from build123d import *

# Parameters (mm, degrees)
BASE_START                                   = 59
BASE_PLATE_DEPTH                             = 5
BOLT_START                                   = 58.8
SKETCH2_R                                    = 1.7
BOLT_HOLES_CABLE_KIDNEY_DEPTH                = 5.4
CHEEK_START                                  = -36
CHEEK_X_DEPTH                                = 6
PIVOT_START                                  = -36
SKETCH4_R                                    = 17
PIVOT_BOSS_X_DEPTH                           = 6
CHEEK_START_2                                = 30
CHEEK_X_2_DEPTH                              = 6
PIVOT_START_2                                = 30
SKETCH6_R                                    = 17
PIVOT_BOSS_X_2_DEPTH                         = 6
JOURNAL_START                                = -37
SKETCH7_R                                    = 7.25
JOURNAL_BORES_DEPTH                          = 74
BACK_START                                   = -54
SKETCH8_W                                    = 72
SKETCH8_H                                    = 60.7
BACK_WALL_DEPTH                              = 4
PINION_START                                 = -55
SKETCH9_W                                    = 9.2
SKETCH9_H                                    = 45
PINION_NOTCH_DEPTH                           = 6
SERVO_START                                  = 0.55
SKETCH10_W                                   = 28.2
SKETCH10_H                                   = 58.7
SKETCH10_W_2                                 = 20.5
SKETCH10_H_2                                 = 41.5
SERVO_BULKHEAD_DEPTH                         = 5
TAB_START                                    = 0.35
SKETCH11_R                                   = 1.7
TAB_BOLT_HOLES_DEPTH                         = 5.4
TAB_START_2                                  = 2.85
TAB_NUT_POCKETS_DEPTH                        = 2.9
BULKHEAD_START                               = 0.35
BULKHEAD_CHAMFER_DEPTH                       = 5.4
HAND_START                                   = 0.35
SKETCH14_W                                   = 21.65
SKETCH14_H                                   = 13.8
HAND_FIX_BAR_OVER_THE_SERVO_WINDOW_SAW_DEPTH = 5.4


with BuildPart() as part:
    # Sketch1 → Base plate (new body)
    with BuildSketch(Plane(origin=(0, 0, 0), x_dir=(1, 0, 0), z_dir=(0, 1, 0)).offset(BASE_START)):
        with BuildLine():
            Line((-30, 54), (30, 54))
            ThreePointArc((30, 54), (34.242640687, 52.242640687), (36, 48))
            Line((36, 48), (36, -20))
            ThreePointArc((36, -20), (33.071067812, -27.071067812), (26, -30))
            Line((26, -30), (-26, -30))
            ThreePointArc((-26, -30), (-33.071067812, -27.071067812), (-36, -20))
            Line((-36, -20), (-36, 48))
            ThreePointArc((-36, 48), (-34.242640687, 52.242640687), (-30, 54))
        make_face()
    extrude(amount=BASE_PLATE_DEPTH)

    # Sketch2 → Bolt holes _ cable kidney (cut)
    with BuildSketch(Plane(origin=(0, 0, 0), x_dir=(1, 0, 0), z_dir=(0, 1, 0)).offset(BOLT_START)):
        with Locations(Location((-26, 44, 0), (0, 0, 90))):
            Circle(SKETCH2_R)
        with Locations(Location((-26, -22, 0), (0, 0, 90))):
            Circle(SKETCH2_R)
        with Locations(Location((26, 44, 0), (0, 0, 90))):
            Circle(SKETCH2_R)
        with Locations(Location((26, -22, 0), (0, 0, 90))):
            Circle(SKETCH2_R)
        with BuildLine():
            ThreePointArc((-35.238044383, 29.568230046), (0, 46), (35.238044383, 29.568230046))
            ThreePointArc((35.238044383, 29.568230046), (34.498503383, 21.115237729), (26.045511066, 21.854778729))
            ThreePointArc((26.045511066, 21.854778729), (0, 34), (-26.045511066, 21.854778729))
            ThreePointArc((-26.045511066, 21.854778729), (-34.498503383, 21.115237729), (-35.238044383, 29.568230046))
        make_face()
    extrude(amount=BOLT_HOLES_CABLE_KIDNEY_DEPTH, mode=Mode.SUBTRACT)


with BuildPart() as bolt_holes_cable_kidney_piece_1:
    # of the separate pieces the step leaves, piece 1, a body of its own (bolt_holes_cable_kidney_pieces)
    add(part.part.solids().sort_by_distance((-36, 59, 20))[0])



with BuildPart() as bolt_holes_cable_kidney_piece_2:
    # of the separate pieces the step leaves, piece 2, a body of its own (bolt_holes_cable_kidney_pieces)
    add(part.part.solids().sort_by_distance((-30, 59, -54))[0])


with BuildPart() as bolt_holes_cable_kidney_piece_1_1:
    add(bolt_holes_cable_kidney_piece_1.part)

    add(bolt_holes_cable_kidney_piece_2.part)  # Cheek -X merges Bolt holes _ cable kidney piece 2
    # Sketch3 → Cheek -X (add)
    with BuildSketch(Plane(origin=(0, 0, 0), x_dir=(0, 0, -1), z_dir=(1, 0, 0)).offset(CHEEK_START)):
        with BuildLine():
            Line((54, 63.8), (-22, 63.8))
            ThreePointArc((-22, 63.8), (-26.242640687, 65.557359313), (-28, 69.8))
            Line((-28, 69.8), (-28, 96.357864376))
            ThreePointArc((-28, 96.357864376), (-27.238795325, 100.1846987), (-25.071067812, 103.428932188))
            Line((-25.071067812, 103.428932188), (-11.622364452, 116.877635548))
            ThreePointArc((-11.622364452, 116.877635548), (-9.843658462, 118.217921148), (-7.764386256, 119.015910864))
            Line((-7.764386256, 119.015910864), (15.334171088, 124.346347174))
            ThreePointArc((15.334171088, 124.346347174), (16.004388899, 124.461463035), (16.683328128, 124.5))
            Line((16.683328128, 124.5), (54, 124.5))
            Line((54, 124.5), (54, 63.8))
        make_face()
    extrude(amount=CHEEK_X_DEPTH)

    # Sketch4 → Pivot boss -X (add)
    with BuildSketch(Plane(origin=(0, 0, 0), x_dir=(0, 0, -1), z_dir=(1, 0, 0)).offset(PIVOT_START)):
        with Locations((-14, 102.5)):
            Circle(SKETCH4_R)
    extrude(amount=PIVOT_BOSS_X_DEPTH)

    # Sketch5 → Cheek _X 2 (add)
    with BuildSketch(Plane(origin=(0, 0, 0), x_dir=(0, 0, -1), z_dir=(1, 0, 0)).offset(CHEEK_START_2)):
        with BuildLine():
            Line((54, 63.8), (-22, 63.8))
            ThreePointArc((-22, 63.8), (-26.242640687, 65.557359313), (-28, 69.8))
            Line((-28, 69.8), (-28, 96.357864376))
            ThreePointArc((-28, 96.357864376), (-27.238795325, 100.1846987), (-25.071067812, 103.428932188))
            Line((-25.071067812, 103.428932188), (-11.622364452, 116.877635548))
            ThreePointArc((-11.622364452, 116.877635548), (-9.843658462, 118.217921148), (-7.764386256, 119.015910864))
            Line((-7.764386256, 119.015910864), (15.334171088, 124.346347174))
            ThreePointArc((15.334171088, 124.346347174), (16.004388899, 124.461463035), (16.683328128, 124.5))
            Line((16.683328128, 124.5), (54, 124.5))
            Line((54, 124.5), (54, 63.8))
        make_face()
    extrude(amount=CHEEK_X_2_DEPTH)

    # Sketch6 → Pivot boss _X 2 (add)
    with BuildSketch(Plane(origin=(0, 0, 0), x_dir=(0, 0, -1), z_dir=(1, 0, 0)).offset(PIVOT_START_2)):
        with Locations((-14, 102.5)):
            Circle(SKETCH6_R)
    extrude(amount=PIVOT_BOSS_X_2_DEPTH)

    # Sketch7 → Journal bores (cut)
    with BuildSketch(Plane(origin=(0, 0, 0), x_dir=(0, 0, -1), z_dir=(1, 0, 0)).offset(JOURNAL_START)):
        with Locations(Location((-14, 102.5, 0), (0, 0, 180))):
            Circle(SKETCH7_R)
    extrude(amount=JOURNAL_BORES_DEPTH, mode=Mode.SUBTRACT)

    # Sketch8 → Back wall (add)
    with BuildSketch(Plane.XY.offset(BACK_START)):
        with Locations((0, 94.15)):
            Rectangle(SKETCH8_W, SKETCH8_H)
    extrude(amount=BACK_WALL_DEPTH)

    # Sketch9 → Pinion notch (cut)
    with BuildSketch(Plane.XY.offset(PINION_START)):
        with Locations((24.85, 103)):
            Rectangle(SKETCH9_W, SKETCH9_H)
    extrude(amount=PINION_NOTCH_DEPTH, mode=Mode.SUBTRACT)

    # Sketch10 → Servo bulkhead (add)
    with BuildSketch(Plane(origin=(0, 0, 0), x_dir=(0, 0, -1), z_dir=(1, 0, 0)).offset(SERVO_START)):
        with Locations((36.1, 93.15)):
            Rectangle(SKETCH10_W, SKETCH10_H)
        with Locations((38.6, 92.15)):
            Rectangle(SKETCH10_W_2, SKETCH10_H_2, mode=Mode.SUBTRACT)
    extrude(amount=SERVO_BULKHEAD_DEPTH)

    # Sketch11 → Tab bolt holes (cut)
    with BuildSketch(Plane(origin=(0, 0, 0), x_dir=(0, 0, -1), z_dir=(1, 0, 0)).offset(TAB_START)):
        with Locations(Location((33.6, 116.9, 0), (0, 0, 180))):
            Circle(SKETCH11_R)
        with Locations(Location((43.6, 116.9, 0), (0, 0, 180))):
            Circle(SKETCH11_R)
        with Locations(Location((33.6, 67.4, 0), (0, 0, 180))):
            Circle(SKETCH11_R)
        with Locations(Location((43.6, 67.4, 0), (0, 0, 180))):
            Circle(SKETCH11_R)
    extrude(amount=TAB_BOLT_HOLES_DEPTH, mode=Mode.SUBTRACT)

    # Sketch12 → Tab nut pockets (cut)
    with BuildSketch(Plane(origin=(0, 0, 0), x_dir=(0, 0, -1), z_dir=(1, 0, 0)).offset(TAB_START_2)):
        Polygon((31.896816706, 119.85), (30.193633412, 116.9), (31.896816706, 113.95), (35.303183294, 113.95), (37.006366588, 116.9), (35.303183294, 119.85), align=None)
        Polygon((41.896816706, 119.85), (40.193633412, 116.9), (41.896816706, 113.95), (45.303183294, 113.95), (47.006366588, 116.9), (45.303183294, 119.85), align=None)
        Polygon((31.896816706, 70.35), (30.193633412, 67.4), (31.896816706, 64.45), (35.303183294, 64.45), (37.006366588, 67.4), (35.303183294, 70.35), align=None)
        Polygon((41.896816706, 70.35), (40.193633412, 67.4), (41.896816706, 64.45), (45.303183294, 64.45), (47.006366588, 67.4), (45.303183294, 70.35), align=None)
    extrude(amount=TAB_NUT_POCKETS_DEPTH, mode=Mode.SUBTRACT)

    # Sketch13 → Bulkhead chamfer (cut)
    with BuildSketch(Plane(origin=(0, 0, 0), x_dir=(0, 0, -1), z_dir=(1, 0, 0)).offset(BULKHEAD_START)):
        Polygon((21.8, 108.5), (21.8, 122.7), (30, 122.7), align=None)
    extrude(amount=BULKHEAD_CHAMFER_DEPTH, mode=Mode.SUBTRACT)

    # Sketch14 → HAND FIX - bar over the servo window saw (cut)
    with BuildSketch(Plane(origin=(0, 0, 0), x_dir=(0, 0, -1), z_dir=(1, 0, 0)).offset(HAND_START)):
        with Locations((39.175, 119.6)):
            Rectangle(SKETCH14_W, SKETCH14_H)
    extrude(amount=HAND_FIX_BAR_OVER_THE_SERVO_WINDOW_SAW_DEPTH, mode=Mode.SUBTRACT)


solid = bolt_holes_cable_kidney_piece_1_1.part
CAD build for the part. Positions are in the model's coordinates, mm. A direction names the side the tool comes from. Coordinates: 2 decimals unless noted, no trailing zeros. Order: outer loops, then holes, each group sorted by start corner. A loop starts at its lowest first (then second) coordinate and runs counter-clockwise, first axis right, second up.
Item 1: Band-saw the part on C-C on x = 17.5. List the corners of the cut face in (y, z).
Check sheet entries:
outline: (59, -54) - (124.5, -54) - (124.5, -50) - (64, -50) - (64, -42.54) - (59, -42.54) - close; (59, -29.15) - (64, -29.15) - (64, 30) - (59, 30) - close
Item 2: Two-plate mould, pull along Z, no slides. Class faces 5 (the face through (4.18, 68.85, -36.17)), 6 (the face through (-18, 64, -46)), 7 (the face through (4.18, 65.9, -36.14)), 8 (the face through (-1, 92, -54)): +Z half, -Z half, draft (parallel to the pull), parting line (faces both ways), or undercut.
Check sheet entries:
face 5: undercut
face 6: draft
face 7: undercut
face 8: -Z half
Item 3: Band-saw the part on A-A on y = 102.5. List the corners of the cut face in (x, z).
Check sheet entries:
outline: (-36, -54) - (20.25, -54) - (20.25, -50) - (5.55, -50) - (5.55, -48.85) - (0.55, -48.85) - (0.55, -50) - (-30, -50) - (-30, 6.75) - (-36, 6.75) - close; (-36, 21.25) - (-30, 21.25) - (-30, 31) - (-36, 31) - close; (0.55, -28.35) - (5.55, -28.35) - (5.55, -22) - (0.55, -22) - close; (29.45, -54) - (36, -54) - (36, 6.75) - (30, 6.75) - (30, -50) - (29.45, -50) - close; (30, 21.25) - (36, 21.25) - (36, 31) - (30, 31) - close
Item 4: Band-saw the part on D-D on z = 14. List the corners of the cut face in (x, y), plus the area to 3 significant figures.
Check sheet entries:
outline: (-36, 59) - (36, 59) - (36, 95.25) - (30, 95.25) - (30, 64) - (-30, 64) - (-30, 95.25) - (-36, 95.25) - close; (-36, 109.75) - (-30, 109.75) - (-30, 119.5) - (-36, 119.5) - close; (30, 109.75) - (36, 109.75) - (36, 119.5) - (30, 119.5) - close
area: 852 mm2
Item 5: Pin check, flat tips, straight feed: pin 1 Ø1.5 at (x, y) = (-15.5, 108) entering from +Z; pin 2 Ø3 at (x, z) = (-26, -44) entering from -Y; pin 3 Ø4 at (x, z) = (4, -41) entering from +Y; pin 4 Ø12 at (x, y) = (-23.5, 67) entering from +Z. Stop position of each tip, or through.
Check sheet entries:
pin 1: stops at z = -50
pin 2: passes through
pin 3: stops at y = 71.4
pin 4: stops at z = 30
Item 6: Band-saw the part on B-B on y = 87.5. List the corners of the cut face in (x, z).
Check sheet entries:
outline: (-36, -54) - (20.25, -54) - (20.25, -50) - (5.55, -50) - (5.55, -48.85) - (0.55, -48.85) - (0.55, -50) - (-30, -50) - (-30, 28) - (-36, 28) - close; (0.55, -28.35) - (5.55, -28.35) - (5.55, -22) - (0.55, -22) - close; (29.45, -54) - (36, -54) - (36, 28) - (30, 28) - (30, -50) - (29.45, -50) - close
Item 7: 3-axis set-ups, long thin cutter, end or side, ignore diameter. For faces 1 (the face through (3, 63.8, -40)), 2 (the face through (25, 80.5, -52)), 3 (the face through (4, 70.35, -34)), 4 (the face through (21, 64, -46)): which of +Z, -Z, +X, -X, +Y, -Y reach the whole face in a straight line?
Check sheet entries:
face 1: -Y
face 2: +Z, -Z, +Y
face 3: none
face 4: +Z, +Y
Item 8: Drill centre lines: L1, parallel to X at y = 78, z = -27.5; L2, parallel to Y at x = 33, z = 14; L3, parallel to X at y = 90, z = -40. Where is each one in solid material? Low to high.
Check sheet entries:
L1: x = -36 to -30, 0.55 to 5.55, 30 to 36
L2: y = 59 to 95.25, 109.75 to 119.5
L3: x = -36 to -30, 30 to 36
